from build123d import *

# Parameters (mm, degrees)
SKETCH1_R           = 19
SKETCH1_R_2         = 6
BOSS_EXTRUDE1_DEPTH = 11
SKETCH2_R           = 8.25
SKETCH2_R_2         = 6
BOSS_EXTRUDE2_DEPTH = 5
SKETCH3_R           = 3.5
BOSS_EXTRUDE3_DEPTH = 5
FILLET1_R           = 3


with BuildPart() as part:
    # Sketch1 → Boss-Extrude1 (new body)
    with BuildSketch(Plane.XY):
        Circle(SKETCH1_R)
        Circle(SKETCH1_R_2, mode=Mode.SUBTRACT)
    extrude(amount=BOSS_EXTRUDE1_DEPTH)

    # Sketch2 → Boss-Extrude2 (add)
    with BuildSketch(Plane.XY.offset(11)):
        Circle(SKETCH2_R)
        Circle(SKETCH2_R_2, mode=Mode.SUBTRACT)
    extrude(amount=BOSS_EXTRUDE2_DEPTH)

    # Sketch3 → Boss-Extrude3 (add)
    # profile 1 of 2: a face of its own
    with BuildSketch(Plane(origin=(0, 0, 0), x_dir=(-1, 0, 0), z_dir=(0, 0, -1))):
        with BuildLine():
            Line((31, 4.5), (31, -4.5))
            Line((31, -4.5), (15.364682716, -11.177053505))
            ThreePointArc((15.364682716, -11.177053505), (19, 0), (15.364682716, 11.177053505))
            Line((15.364682716, 11.177053505), (31, 4.5))
        make_face()
        with Locations((24, 0)):
            Circle(SKETCH3_R, mode=Mode.SUBTRACT)
    # profile 2 of 2: a face of its own
    with BuildSketch(Plane(origin=(0, 0, 0), x_dir=(-1, 0, 0), z_dir=(0, 0, -1))):
        with BuildLine():
            Line((-15.364682716, -11.177053505), (-31, -4.5))
            Line((-31, -4.5), (-31, 4.5))
            Line((-31, 4.5), (-15.364682716, 11.177053505))
            ThreePointArc((-15.364682716, 11.177053505), (-19, 0), (-15.364682716, -11.177053505))
        make_face()
        with Locations((-24, 0)):
            Circle(SKETCH3_R, mode=Mode.SUBTRACT)
    extrude(amount=-BOSS_EXTRUDE3_DEPTH)

    # Fillet1
    fillet1_edges = [part.edges().sort_by_distance(p)[0] for p in [
        (31, -4.5, 2.5),
        (31, 4.5, 2.5),
        (-31, 4.5, 2.5),
        (-31, -4.5, 2.5),
    ]]
    fillet(fillet1_edges, radius=FILLET1_R)


solid = part.part
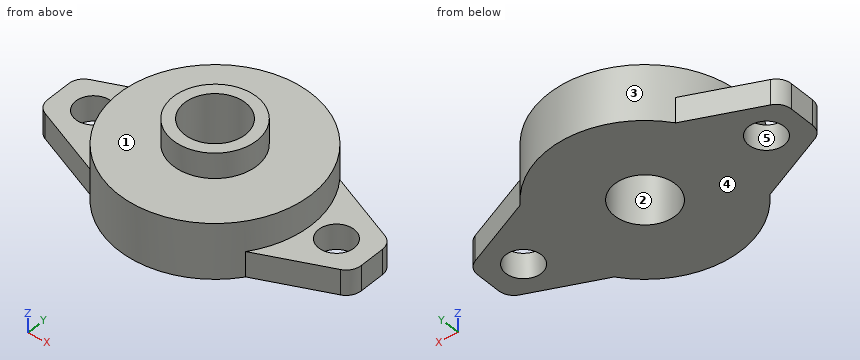
Geometry: final body of the model. Coordinates: model frame, mm. Face numbers are marked on the shaded views. A direction names the side the tool comes from. Coordinates: 2 decimals unless noted, no trailing zeros. Order: outer loops, then holes, each group sorted by start corner. A loop starts at its lowest first (then second) coordinate and runs counter-clockwise, first axis right, second up. Notation, with made-up numbers: M -11.5,-14 L -6.5,-14 A23 cw -6.5,10 Z; hole C 45,18 d8. An arc over 180 degrees is marked long. One line per question, with ' | ' between items. Start each with the question number.
Item 1: Pin query (flat end, axial travel): pin 1 Ø1.5 at (x, z) = (4.5, 6.5) entering from +Y; pin 2 Ø1 at (y, z) = (13, 9) entering from -X; pin 3 Ø3 at (x, y) = (-13, 3) entering from +Z. Return the tip coordinate at first contact, or that it passes through.
Item 2: Cut plane B-B, the plane z = 4. Return the cut outline in (x, y).
Item 3: Cut plane A-A, the plane x = 0. Return the cut outline in (y, z), then the cut area to 4 significant figures.
Item 4: Ray query, probe 1 along Y at (x, z) = (0, 7.25); probe 2 along X at (y, z) = (-5, 11.5); probe 3 along Z at (x, y) = (-7.5, 15). Return the intervals inside material, ascending. Write a range as [from, to].
Item 5: Set-up query: the marked faces 1 and 2. Return all of +Z, -Z, +X, -X, +Y, -Y with unobstructed straight access to the full face (end or side cutting, diameter ignored); none if empty.
Item 6: Cut plane C-C, the plane y = 0. Return the cut outline in (x, z).
Item 7: Draft query along Y for the marked faces 3, 4 and 5. Return one class per face: released by +Y, released by -Y, zero draft, split by the parting line, or undercut.
Item 8: Cut plane D-D, the plane z = 14. Return the cut outline in (x, y), then the cut area to 3 significant figures.
A:
1) pin 1: stops at y = 18.63 | pin 2: stops at x = -14.31 | pin 3: stops at z = 11
2) outline: M -31,-2.52 A3 ccw -29.18,-5.28 L -15.36,-11.18 A19 ccw 15.36,-11.18 L 29.18,-5.28 A3 ccw 31,-2.52 L 31,2.52 A3 ccw 29.18,5.28 L 15.36,11.18 A19 ccw -15.36,11.18 L -29.18,5.28 A3 ccw -31,2.52 Z; hole C -24,0 d7; hole C 0,0 d12; hole C 24,0 d7
3) outline: M -19,0 L -6,0 L -6,16 L -8.25,16 L -8.25,11 L -19,11 Z; M 6,0 L 19,0 L 19,11 L 8.25,11 L 8.25,16 L 6,16 Z | area: 308.5 mm2
4) probe 1: y = [-19, -6], [6, 19] | probe 2: x = [-6.56, -3.32], [3.32, 6.56] | probe 3: z = [0, 11]
5) face 1: +Z | face 2: +Z, -Z
6) outline: M -31,0 L -27.5,0 L -27.5,5 L -31,5 Z; M -20.5,0 L -6,0 L -6,16 L -8.25,16 L -8.25,11 L -19,11 L -19,5 L -20.5,5 Z; M 6,0 L 20.5,0 L 20.5,5 L 19,5 L 19,11 L 8.25,11 L 8.25,16 L 6,16 Z; M 27.5,0 L 31,0 L 31,5 L 27.5,5 Z
7) face 3: split by the parting line | face 4: zero draft | face 5: undercut
8) outline: C 0,0 d16.5; hole C 0,0 d12 | area: 101 mm2
